Here's how the part is built. I have some questions about the finished solid (model axes, mm). Round coordinates to 2 decimals unless told otherwise and drop trailing zeros. Loops run counter-clockwise (first coordinate to the right, second up) from the corner with the lowest first, then second, coordinate; pieces in that order, holes last. Notation, with made-up numbers: (-15, -29) - (3, -29) arc R34 ccw to (3, 6) - close; hole circle Ø10 at (79.5, 44). An arc over 180 degrees is marked (long way). Answer as a JSON object with one key per item and string values. Group by question number.
1) I want a section at A-A, the plane x = 0. Please give me the cut outline in (y, z).
2) If I drill on line 1 along Y through (x, z) = (0, 2.55); line 2 along Y through (x, z) = (-20, 3.3); line 3 along X through (y, z) = (39.5, 1.45), over which ranges is the centre line in solid material (lowest first)? Write a range as [from, to].
3) If we mould it in two halves opening along X, with no side actions, what happens to faces 1 (the face through (30, -1, 2)), 2 (the face through (0, -50, 2)), 3 (the face through (21.425, -37.766, 2.535)), 4 (the face through (-18.575, -37.766, 2.535))? For each: pulls with the +X half, pulls with the -X half, needs draft (parallel to the pull), parting line crosses it, or undercut.
4) I want a section at B-B, the plane y = 40. Please give me the cut outline in (x, z), then the cut area to 3 significant figures.
5) Will these pins go through, and if not, where does the flat tip stop? P1, Ø3, axis at x = 0, y = 32.5, coming from the +Z side; P2, Ø12, axis at x = -20, y = -6, coming from the -Z side.
from build123d import *

# Parameters (mm, degrees)
SKETCH_W        = 60
SKETCH_H        = 100
PAD_DEPTH       = 5
SKETCH001_R     = 2.65
POCKET_DEPTH    = 5
FILLET_R        = 11
SKETCH002_R     = 2.5
POCKET001_DEPTH = 5


with BuildPart() as part:
    # Sketch → Pad (new body)
    with BuildSketch(Plane.XY):
        Rectangle(SKETCH_W, SKETCH_H)
    extrude(amount=PAD_DEPTH)

    # Sketch001 (on Face6 of Pad) → Pocket (cut)
    with BuildSketch(Plane.XY.offset(5)):
        with Locations((-20, 40)):
            Circle(SKETCH001_R)
        with Locations((20, 40)):
            Circle(SKETCH001_R)
        with Locations((-20, -40)):
            Circle(SKETCH001_R)
        with Locations((20, -40)):
            Circle(SKETCH001_R)
    extrude(amount=-POCKET_DEPTH, mode=Mode.SUBTRACT)

    # Fillet
    fillet_edges = [part.edges().sort_by_distance(p)[0] for p in [
        (30, 50, 2.5),
        (30, -50, 2.5),
        (-30, 50, 2.5),
        (-30, -50, 2.5),
    ]]
    fillet(fillet_edges, radius=FILLET_R)

    # Sketch002 (on Face5 of Fillet) → Pocket001 (cut)
    with BuildSketch(Plane.XY.offset(5)):
        with Locations((0, 32.5)):
            Circle(SKETCH002_R)
        with Locations((0, -32.5)):
            Circle(SKETCH002_R)
    extrude(amount=-POCKET001_DEPTH, mode=Mode.SUBTRACT)


solid = part.part
Outcome:
{
 "1": {"outline": "(-50, 0) - (-35, 0) - (-35, 5) - (-50, 5) - close; (-30, 0) - (30, 0) - (30, 5) - (-30, 5) - close; (35, 0) - (50, 0) - (50, 5) - (35, 5) - close"},
 "2": {"line 1": "[-50, -35], [-30, 30], [35, 50]", "line 2": "[-49.95, -42.65], [-37.35, 37.35], [42.65, 49.95]", "line 3": "[-29.99, -22.6], [-17.4, 17.4], [22.6, 29.99]"},
 "3": {"face 1": "pulls with the +X half", "face 2": "needs draft", "face 3": "undercut", "face 4": "undercut"},
 "4": {"outline": "(-29.95, 0) - (-22.65, 0) - (-22.65, 5) - (-29.95, 5) - close; (-17.35, 0) - (17.35, 0) - (17.35, 5) - (-17.35, 5) - close; (22.65, 0) - (29.95, 0) - (29.95, 5) - (22.65, 5) - close", "area": "247 mm^2"},
 "5": {"P1": "through", "P2": "z = 0"}
}
